Input: part model. Units: mm. Frame: model coordinates. Give positions to 0.01 mm unless a question says otherwise; leave off trailing zeros. Loops run counter-clockwise (first coordinate to the right, second up) from the corner with the lowest first, then second, coordinate; pieces in that order, holes last. Notation, with made-up numbers: M 32,4.25 L 36,4.25 A18 cw 36,20.25 Z; hole C 24,86 d10. An arc over 180 degrees is marked long. One line per item, written item: value. Start each with the question number.
(1) Section B-B on x = 0. Output: boundary loops of the cut face in (y, z).
(2) Pin query (flat end, axial travel): P1, Ø4, axis at y = 30, z = -3, coming from the +X side; P2, Ø0.9, axis at x = -1, y = 40.5, coming from the +Z side; P3, Ø1.5, axis at y = 8.5, z = -3.5, coming from the -X side. Return the tip coordinate at first contact, or that it passes through.
(3) Section A-A on y = 0. Output: boundary loops of the cut face in (x, z), plus the area to 4 significant figures.
(4) Ray query, line 1 along Y through (x, z) = (0, -4.1); line 2 along X through (y, z) = (0, 2.2); line 3 along Y through (x, z) = (-1, -3.25). Return the intervals inside material, ascending. Write a range as from..to.
```python
from build123d import *

# Parameters (mm, degrees)
F0_R          = 41.25
F0_R_2        = 40.25
F1_DEPTH      = 3
F1_DEPTH_BACK = 1
F0_R_3        = 38.75
F2_DEPTH      = 5
F3_S5_R       = 40.25
F3_T6_DEPTH   = 60
F3_S11_R      = 40.25
F3_T12_DEPTH  = 58
F4_R          = 41.25
F4_R_2        = 40.25
F5_DEPTH      = 1
F7_END_RADIUS = 41.25
F6_W          = 10
F6_H          = 3
F7_REACH      = 51.6913065089


# Not quite as in the source:
# - a fillet or chamfer that OpenCascade refuses, or shapes differently, is made with other operations: its cross-section is extruded or revolved along the edge and cut away or added


with BuildPart() as f1:
    # F0 (on Top) → F1 (new body, two sides)
    with BuildSketch(Plane.XY) as f1_sk:
        Circle(F0_R)
        Circle(F0_R_2, mode=Mode.SUBTRACT)
    extrude(amount=F1_DEPTH)
    extrude(f1_sk.sketch, amount=-F1_DEPTH_BACK)

    # F0 (on Top) → F2 (join)
    with BuildSketch(Plane.XY):
        Circle(F0_R_2)
        Circle(F0_R_3, mode=Mode.SUBTRACT)
    extrude(amount=-F2_DEPTH)

    # F3: chamfer of 1.5 on 2 edges, made by hand


with BuildPart() as f3_tool2:
    # F3_s3 → F3_t4 (revolve)
    with BuildSketch(Plane.XZ):
        Polygon((41.25, 0.5), (39.75, -1), (41.25, -1), align=None)
    revolve(axis=Axis((0, 0, -1), (0, 0, 1)))

    # F3_s5 → F3_t6 (cut, symmetric)
    with BuildSketch(Plane.XY.offset(-0.3)):
        Circle(F3_S5_R)
    extrude(amount=F3_T6_DEPTH, both=True, mode=Mode.SUBTRACT)


with BuildPart() as f1_1:
    add(f1.part)

    # F3_t1: cut F3_tool2
    add(f3_tool2.part, mode=Mode.SUBTRACT)


with BuildPart() as f3_tool8:
    # F3_s9 → F3_t10 (revolve)
    with BuildSketch(Plane.XZ):
        Polygon((40.25, 0), (38.75, -1.5), (38.75, 0), align=None)
    revolve(axis=Axis((0, 0, 0), (0, 0, 1)))

    # F3_s11 → F3_t12 (intersect, symmetric)
    with BuildSketch(Plane.XY.offset(-0.8)):
        Circle(F3_S11_R)
    extrude(amount=F3_T12_DEPTH, both=True, mode=Mode.INTERSECT)


with BuildPart() as f1_2:
    add(f1_1.part)

    # F3_t7: cut F3_tool8
    add(f3_tool8.part, mode=Mode.SUBTRACT)

    # F4 (on face) → F5 (join)
    with BuildSketch(Plane(origin=(0, 0, -5), x_dir=(1, 0, 0), z_dir=(0, 0, -1))):
        Circle(F4_R)
        Circle(F4_R_2, mode=Mode.SUBTRACT)
    extrude(amount=-F5_DEPTH)

    f7_end = (Plane(origin=(0, 0, 1.75), x_dir=(-1, 0, 0), z_dir=(0, 0, -1)) * Cylinder(F7_END_RADIUS, 337.2757510104, mode=Mode.PRIVATE)).faces().sort_by_distance((-41.25, 0, 1.75))[0]
    # F6 (on Front) → F7 (cut, up to the whole of a round face its end follows)
    with BuildSketch(Plane.XZ):
        with Locations((0, 1.5)):
            Rectangle(F6_W, F6_H)
    f7_long = extrude(amount=-F7_REACH, mode=Mode.PRIVATE)
    add(split(f7_long, bisect_by=f7_end, keep=Keep.BOTTOM, mode=Mode.PRIVATE), mode=Mode.SUBTRACT)


solid = f1_2.part
```
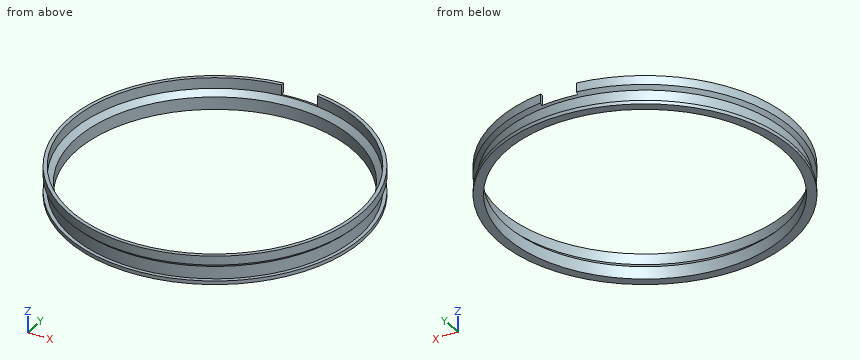
Output values:
1. outline: M -41.25,-5 L -38.75,-5 L -38.75,-1.5 L -40.25,0 L -40.25,3 L -41.25,3 L -41.25,0.5 L -40.25,-0.5 L -40.25,-4 L -41.25,-4 Z; M 38.75,-5 L 41.25,-5 L 41.25,-4 L 40.25,-4 L 40.25,-0.5 L 40.75,0 L 40.25,0 L 38.75,-1.5 Z
2. P1: stops at x = 30.04
2. P2: stops at z = 0
2. P3: stops at x = -40.48
3. outline: M -41.25,-5 L -38.75,-5 L -38.75,-1.5 L -40.25,0 L -40.25,3 L -41.25,3 L -41.25,0.5 L -40.25,-0.5 L -40.25,-4 L -41.25,-4 Z; M 38.75,-5 L 41.25,-5 L 41.25,-4 L 40.25,-4 L 40.25,-0.5 L 41.25,0.5 L 41.25,3 L 40.25,3 L 40.25,0 L 38.75,-1.5 Z
3. area: 20.75 mm²
4. line 1: y = -41.25..-38.75, 38.75..41.25
4. line 2: x = -41.25..-40.25, 40.25..41.25
4. line 3: y = -40.24..-38.74, 38.74..40.24
